```python
from build123d import *

# Parameters (mm, degrees)
F0_R          = 3.9
F0_W          = 5
F0_H          = 30
F1_DEPTH      = 60
F2_W          = 20.1
F2_H          = 40.1
F2_R          = 2.25
F3_DEPTH      = 54.801
F5_W          = 34.2169012874
F5_H          = 48
F6_DEPTH      = 67.901
F6_DEPTH_BACK = 67.901
F7_R          = 5
F9_R          = 1.35
F10_DEPTH     = 7.901


# Not quite as in the source:
# - a pattern or mirror of a feature is missing from the dataset's text; its kind, count and spacing are read off the source's solid


with BuildPart() as f1:
    # F0 (on Top) → F1 (new body)
    with BuildSketch(Plane.XY):
        with BuildLine():
            ThreePointArc((-52.3022123868, 6.1240310078), (-55.0816748297, 1.717761124), (-60, 0))
            Line((-60, 0), (-47.43019491, 0))
            ThreePointArc((-47.43019491, 0), (-51.3430043252, 1.8871359682), (-52.3022123868, 6.1240310078))
        make_face()
        Polygon((-47.43019491, 0), (-60, 0), (-60, -5), (-18.1, -5), (-13.1, -5), (60, -5), (60, 0), (47.43019491, 0), align=None)
        with BuildLine():
            Line((-60, -5), (-60, 0))
            ThreePointArc((-60, 0), (-61.846439606, 0.218811239), (-63.5905952277, 0.8631238528))
            ThreePointArc((-63.5905952277, 0.8631238528), (-60.9689691941, -1.5623919871), (-60, -5))
        make_face()
        with BuildLine():
            ThreePointArc((-63.5905952277, 0.8631238528), (-61.846439606, 0.218811239), (-60, 0))
            ThreePointArc((-60, 0), (-55.0816748297, 1.717761124), (-52.3022123868, 6.1240310078))
            ThreePointArc((-52.3022123868, 6.1240310078), (-52.1507158879, 7.0062780479), (-52.1, 7.9))
            ThreePointArc((-52.1, 7.9), (-64.125790694, 14.6370506269), (-63.5905952277, 0.8631238528))
        make_face()
        with Locations((-60, 7.9)):
            Circle(F0_R, mode=Mode.SUBTRACT)
        with BuildLine():
            ThreePointArc((52.3022123868, 6.1240310078), (51.3430043252, 1.8871359682), (47.43019491, 0))
            Line((47.43019491, 0), (60, 0))
            ThreePointArc((60, 0), (55.0816748297, 1.717761124), (52.3022123868, 6.1240310078))
        make_face()
        with Locations((-15.6, -20)):
            Rectangle(F0_W, F0_H)
        with BuildLine():
            ThreePointArc((63.5905952277, 0.8631238528), (61.846439606, 0.218811239), (60, 0))
            Line((60, 0), (60, -5))
            ThreePointArc((60, -5), (60.9689691941, -1.5623919871), (63.5905952277, 0.8631238528))
        make_face()
        with BuildLine():
            ThreePointArc((52.3022123868, 6.1240310078), (55.0816748297, 1.717761124), (60, 0))
            ThreePointArc((60, 0), (61.846439606, 0.218811239), (63.5905952277, 0.8631238528))
            ThreePointArc((63.5905952277, 0.8631238528), (66.7370506269, 3.774209306), (67.9, 7.9))
            ThreePointArc((67.9, 7.9), (59.1062780479, 15.7492841121), (52.3022123868, 6.1240310078))
        make_face()
        with Locations((60, 7.9)):
            Circle(F0_R, mode=Mode.SUBTRACT)
    extrude(amount=F1_DEPTH)

    # F2 (on face) → F3 (cut, through all)
    with BuildSketch(Plane.YZ.offset(-13.1)):
        with Locations((-21.95, 30)):
            Rectangle(F2_W, F2_H)
        with Locations((-26.95, 54.75)):
            Circle(F2_R)
        with Locations((-16.95, 54.75)):
            Circle(F2_R)
        with Locations((-16.95, 5.25)):
            Circle(F2_R)
        with Locations((-26.95, 5.25)):
            Circle(F2_R)
    extrude(amount=-F3_DEPTH, mode=Mode.SUBTRACT)

    # F5 (on Right) → F6 (cut, two sides)
    with BuildSketch(Plane.YZ) as f6_sk:
        with Locations((17.1084506437, 30)):
            Rectangle(F5_W, F5_H)
    extrude(amount=-F6_DEPTH, mode=Mode.SUBTRACT)
    extrude(f6_sk.sketch, amount=F6_DEPTH_BACK, mode=Mode.SUBTRACT)

    # F7
    f7_edges = [f1.edges().sort_by_distance(p)[0] for p in [
        (-13.1, -5, 30),
        (-18.1, -5, 30),
    ]]
    fillet(f7_edges, radius=F7_R)

    # F9 (on offset) → F10 (cut, through all)
    with BuildSketch(Plane.YZ.offset(60)):
        with Locations((7.9, 57)):
            Circle(F9_R)
        with Locations((7.9, 3)):
            Circle(F9_R)
    f10 = extrude(amount=F10_DEPTH, mode=Mode.SUBTRACT)

    # F10_copies: F10 across plane
    add(f10.mirror(Plane(origin=(-5e-06, 0, 0), x_dir=(0, 0, -1), z_dir=(-1, 0, 0))), mode=Mode.SUBTRACT)


solid = f1.part
```
Input: part model. Units: mm. Frame: model coordinates. A direction names the side the tool comes from. Round coordinates to 2 decimals unless told otherwise and drop trailing zeros. Order: outer loops, then holes, each group sorted by start corner. A loop starts at its lowest first (then second) coordinate and runs counter-clockwise, first axis right, second up. Notation, with made-up numbers: (43, -20.5) - (96, -20.5) arc R20 cw to (96, -4.5) - close; hole circle Ø10 at (-17, 70.25). An arc over 180 degrees is marked (long way). Answer in a Markdown table with one row per item.
Item 1: Line query: line 1 (X direction, y = 8, z = 55.5); line 2 (Z direction, x = -16.35, y = -16.95); line 3 (Y direction, x = -15, z = 5). Output: solid intervals per line, ascending.
Model answer:
| item | result |
|---|---|
| line 1 | x = -67.9 to -63.9, -56.1 to -52.1, 52.1 to 56.1, 63.9 to 67.9 |
| line 2 | z = 0 to 3, 7.5 to 9.95, 50.05 to 52.5, 57 to 60 |
| line 3 | y = -35 to -29.19, -24.71 to -19.19, -14.71 to 0 |
Item 2: Pin query (flat end, axial travel): pin 1 (5 mm diameter, centred on x = -35.5, z = 24, fed in from +Y); pin 2 (1.6 mm diameter, centred on y = 7.9, z = 3, fed in from -X); pin 3 (20 mm diameter, centred on y = -19.5, z = 24, fed in from +X). Return the tip coordinate at first contact, or that it passes through.
Model answer:
| item | result |
|---|---|
| pin 1 | stops at y = 0 |
| pin 2 | stops at x = -56.18 |
| pin 3 | stops at x = -13.07 |
Item 3: Section query B-B (z = 36). Return the cut outline in (x, y).
Model answer:
| item | result |
|---|---|
| outline | (-62.3, 0) arc R6.58 cw to (-60, -5) - (-23.1, -5) arc R5 cw to (-18.1, -10) - (-18.1, -11.9) - (-13.1, -11.9) - (-13.1, -10) arc R5 cw to (-8.1, -5) - (60, -5) arc R6.58 cw to (62.3, 0) - close; (-18.1, -35) - (-13.1, -35) - (-13.1, -32) - (-18.1, -32) - close |
Item 4: Mould query, pull axis X, two halves, no side actions, for faces 1 (the flat face through (1, 0, 30)), 2 (the flat face through (-13.1, -11.6, 22.9)), 3 (the cylindrical face through (-65.751, 9.147, 56.483)). Classes: released by +X, released by -X, zero draft, split by the parting line, or undercut.
Model answer:
| item | result |
|---|---|
| face 1 | undercut |
| face 2 | released by +X |
| face 3 | zero draft |
Item 5: Section query C-C (y = -22.5). Return the cut outline in (x, z), then the cut area to 3 significant figures.
Model answer:
| item | result |
|---|---|
| outline | (-18.1, 0) - (-13.1, 0) - (-13.1, 9.95) - (-18.1, 9.95) - close; (-18.1, 50.05) - (-13.1, 50.05) - (-13.1, 60) - (-18.1, 60) - close |
| area | 99.5 mm² |
Item 6: Reachability of faces 4 (the flat face through (-16, -32, 30)), 5 (the flat face through (-58, 4, 6)), 6 (the cylindrical face through (51.382, 1.937, 56.958)) from +Z, -Z, +X, -X, +Y, -Y: full face, straight path, thin tool, end or side. Return the list, or none.
Model answer:
| item | result |
|---|---|
| face 4 | +X, -X |
| face 5 | +X, -X, +Y |
| face 6 | +Z, -Z |
Item 7: Section query D-D (x = 21.5). Return the cut outline in (y, z).
Model answer:
| item | result |
|---|---|
| outline | (-5, 0) - (0, 0) - (0, 60) - (-5, 60) - close |
Item 8: Section query A-A (y = -16.95). Return the cut outline in (x, z), then the cut area to 3 significant figures.
Model answer:
| item | result |
|---|---|
| outline | (-18.1, 0) - (-13.1, 0) - (-13.1, 3) - (-18.1, 3) - close; (-18.1, 7.5) - (-13.1, 7.5) - (-13.1, 9.95) - (-18.1, 9.95) - close; (-18.1, 50.05) - (-13.1, 50.05) - (-13.1, 52.5) - (-18.1, 52.5) - close; (-18.1, 57) - (-13.1, 57) - (-13.1, 60) - (-18.1, 60) - close |
| area | 54.5 mm² |
